Input: part model. Units: mm. Frame: model coordinates. A direction names the side the tool comes from. Coordinates: 2 decimals unless noted, no trailing zeros. Loops run counter-clockwise (first coordinate to the right, second up) from the corner with the lowest first, then second, coordinate; pieces in that order, holes last. Notation, with made-up numbers: (33, 6) -> (57, 6) arc R21 cw to (57, 12) -> close; hole circle Ø6 at (52, 50.5). An arc over 180 degrees is marked (long way). Put each result on its own line as item: value. Start each with the question number.
1) Cut plane D-D (y = -5). Return the cut outline in (x, z).
2) Cut plane A-A (x = 61.5). Return the cut outline in (y, z) (3 decimals), plus the area to 3 significant figures.
3) Cut plane C-C (y = -30.5). Return the cut outline in (x, z).
4) Contact query for flat-ended pins moving along their axis: P1, Ø1, axis at x = 21.5, z = 5, coming from the +Y side (3 decimals); P2, Ø3.5, axis at y = 29.5, z = 1.5, coming from the -X side; P3, Ø16.5, axis at x = 32, y = -58.5, coming from the +Z side. Output: stop coordinate, or through.
5) Set-up query: faces 1 (the flat face through (49, 21, 6.6)), 2 (the flat face through (49, -57, -8.4)), 3 (the cylindrical face through (14.79, 25.603, 0.993)), 4 (the flat face through (49.3, -42.195, -1.54)), 5 (the cylindrical face through (48.8, -12.6, 15.3)). Return all of +Z, -Z, +X, -X, +Y, -Y with unobstructed straight access to the full face (end or side cutting, diameter ignored); none if empty.
6) Pull-direction query (Y, two-part tool) for faces 6 (the flat face through (100, -11, 10)), 7 (the cylindrical face through (85.21, 25.715, 1.019)), 8 (the cylindrical face through (50.28, 27.94, 0.05)); classes: pulls with the +Y half, pulls with the -Y half, needs draft (parallel to the pull), parting line crosses it, or undercut.
7) Cut plane B-B (x = 78). Return the cut outline in (y, z), plus the area to 3 significant figures.
8) Material intervals for L1, parallel to Z at x = 30.5, y = -60; L2, parallel to Z at x = 77.5, y = -12.5; L3, parallel to Y at x = 74, z = 10.75, sorted ascending.
from build123d import *

# Parameters (mm, degrees)
F1_DEPTH  = 100
F2_SIZE   = 10
F3_R      = 3.5
F4_DEPTH  = 30
F5_R      = 3.6
F6_DEPTH  = 30
F7_R      = 1.125
F8_DEPTH  = 40
F11_DEPTH = 93


# Not quite as in the source:
# - a feature names something its author has since deleted; it is built from what else it names


with BuildPart() as f1:
    # F0 (on Right) → F1 (new body)
    with BuildSketch(Plane.YZ):
        with BuildLine():
            Line((25.5061486276, -1.4), (25.8561486276, -1.4))
            ThreePointArc((25.8561486276, -1.4), (32.4222243139, -0.9859028724), (27.1219938253, 2.9118378984))
            Line((27.1219938253, 2.9118378984), (23.5061486276, 6.6))
            Line((23.5061486276, 6.6), (18.2925903906, 6.6))
            Line((18.2925903906, 6.6), (10.6041878433, 11.6))
            Line((10.6041878433, 11.6), (-34.5898121567, 11.6))
            Line((-34.5898121567, 11.6), (-49.5898121567, -8.4))
            Line((-49.5898121567, -8.4), (-64.3958121567, -8.4))
            Line((-64.3958121567, -8.4), (-64.3958121567, -11.4))
            Line((-64.3958121567, -11.4), (-49.5898121567, -11.4))
            Line((-49.5898121567, -11.4), (-34.5898121567, 8.6))
            Line((-34.5898121567, 8.6), (10.6041878433, 8.6))
            Line((10.6041878433, 8.6), (15.6041878433, 3.6))
            Line((15.6041878433, 3.6), (20.6041878433, 3.6))
            Line((20.6041878433, 3.6), (25.5061486276, -1.4))
        make_face()
        with BuildLine():
            Line((-34.5898121567, 11.6), (10.6041878433, 11.6))
            ThreePointArc((10.6041878433, 11.6), (-11.9928121567, 18.3015086266), (-34.5898121567, 11.6))
        make_face()
    extrude(amount=F1_DEPTH)

    # F2
    f2_edges = [f1.edges().sort_by_distance(p)[0] for p in [
        (100, -64.395812, -9.9),
        (0, -64.395812, -9.9),
    ]]
    chamfer(f2_edges, length=F2_SIZE)

    # F3 (on face) → F4 (cut)
    with BuildSketch(Plane.YZ.offset(100)):
        with Locations((29.0639516141, 0)):
            Circle(F3_R)
    extrude(amount=-F4_DEPTH, mode=Mode.SUBTRACT)

    # F5 (on face) → F6 (cut)
    with BuildSketch(Plane(origin=(0, 0, 0), x_dir=(0, -1, 0), z_dir=(-1, 0, 0))):
        with Locations((-29.0639516141, 0)):
            Circle(F5_R)
    extrude(amount=-F6_DEPTH, mode=Mode.SUBTRACT)

    # F7 (on face) → F8 (cut, through all)
    with BuildSketch(Plane.YZ.offset(70)):
        with Locations((29.0639516141, 0)):
            Circle(F7_R)
    extrude(amount=-F8_DEPTH, mode=Mode.SUBTRACT)

    # F10 (on offset) → F11 (cut)
    with BuildSketch(Plane(origin=(3, 0, 0), x_dir=(0, -1, 0), z_dir=(-1, 0, 0))):
        with BuildLine():
            Line((-7.3898630986, 8.6), (31.992161455, 8.6))
            ThreePointArc((31.992161455, 8.6), (12.3011491782, 15.3028562463), (-7.3898630986, 8.6))
        make_face()
    extrude(amount=-F11_DEPTH, mode=Mode.SUBTRACT)


solid = f1.part
Results found:
1. outline: (0, 8.6) -> (3, 8.6) -> (3, 14.47) -> (96, 14.47) -> (96, 8.6) -> (100, 8.6) -> (100, 17.71) -> (0, 17.71) -> close
2. outline: (-64.396, -11.4) -> (-49.59, -11.4) -> (-34.59, 8.6) -> (-31.992, 8.6) arc R32.275 cw to (7.39, 8.6) -> (10.604, 8.6) -> (15.604, 3.6) -> (20.604, 3.6) -> (25.506, -1.4) -> (25.856, -1.4) arc R3.5 ccw (long way) to (27.122, 2.912) -> (23.506, 6.6) -> (18.293, 6.6) -> (10.604, 11.6) arc R41.448 ccw to (-34.59, 11.6) -> (-49.59, -8.4) -> (-64.396, -8.4) -> close; hole circle Ø2.25 at (29.064, 0)
2. area: 350 mm2
3. outline: (0, 8.6) -> (3, 8.6) -> (3, 9.68) -> (96, 9.68) -> (96, 8.6) -> (100, 8.6) -> (100, 13.94) -> (0, 13.94) -> close
4. P1: stops at y = 25.565
4. P2: stops at x = 30
4. P3: stops at z = -8.4
5. face 1: +Z, +X, -X, +Y
5. face 2: +Z, +X, -X, -Y
5. face 3: -X, +Y
5. face 4: -Z, +X, -X
5. face 5: -Z
6. face 6: needs draft
6. face 7: pulls with the +Y half
6. face 8: undercut
7. outline: (-64.4, -11.4) -> (-49.59, -11.4) -> (-34.59, 8.6) -> (-31.99, 8.6) arc R32.27 cw to (7.39, 8.6) -> (10.6, 8.6) -> (15.6, 3.6) -> (20.6, 3.6) -> (25.51, -1.4) -> (25.86, -1.4) arc R3.5 cw to (27.12, 2.91) -> (23.51, 6.6) -> (18.29, 6.6) -> (10.6, 11.6) arc R41.45 ccw to (-34.59, 11.6) -> (-49.59, -8.4) -> (-64.4, -8.4) -> close
7. area: 315 mm2
8. L1: z = -11.4 to -8.4
8. L2: z = 15.3 to 18.3
8. L3: y = -35.23 to -28.83, 4.23 to 11.91
